The figure shows three views and two pictorial views of one solid part (mm, origin at its lowest corner). Answer the questions. A direction names the side the tool comes from. Give positions to 0.01 mm unless a question says otherwise; leave off trailing zeros. Order: outer loops, then holes, each group sorted by start corner. A loop starts at its lowest first (then second) coordinate and runs counter-clockwise, first axis right, second up. Notation, with made-up numbers: (-23.5, 23.25) - (5.5, 23.25) arc R19 cw to (5.5, 57.25) - close; hole circle Ø2 at (-22, 21). An arc over 180 degrees is marked (long way). Use a Markdown table: item, result. Add a question column.
1. Which of the six approach directions +Z, -Z, +X, -X, +Y, -Y give full straight-line access (tool end or side, diameter ignored) to the marked faces 4 and 5?
2. A cutting plane is placed at B-B on z = 154. Determine the outline of the cut face in (x, y), and give its area (3 significant figures).
3. A cutting plane is placed at A-A on x = 100. Determine the outline of the cut face in (y, z).
4. Flat-ended cylindrical pins translate along their axes: P1, Ø15, axis at x = 100, y = 330, coming from the +Z side; P2, Ø22.5, axis at x = 580, y = 50, coming from the -Z side. Find the tip coordinate at first contact, or state that the pin passes through.
5. For a pull along Z with two mould halves and no side action, classify the marked faces 1, 2 and 3 as released by +Z, released by -Z, zero draft, split by the parting line, or undercut.
6. Consider L1, parallel to Y at x = 100, z = 7; L2, parallel to Y at x = 340, z = 370; L3, parallel to Z at x = 312, y = 213.5. Determine where each line is inside the solid, lowest interval first.
7. A cutting plane is placed at C-C on y = 286.5. Determine the outline of the cut face in (x, z), and give its area (3 significant figures).
8. A cutting plane is placed at D-D on x = 204.5. Determine the outline of the cut face in (y, z).
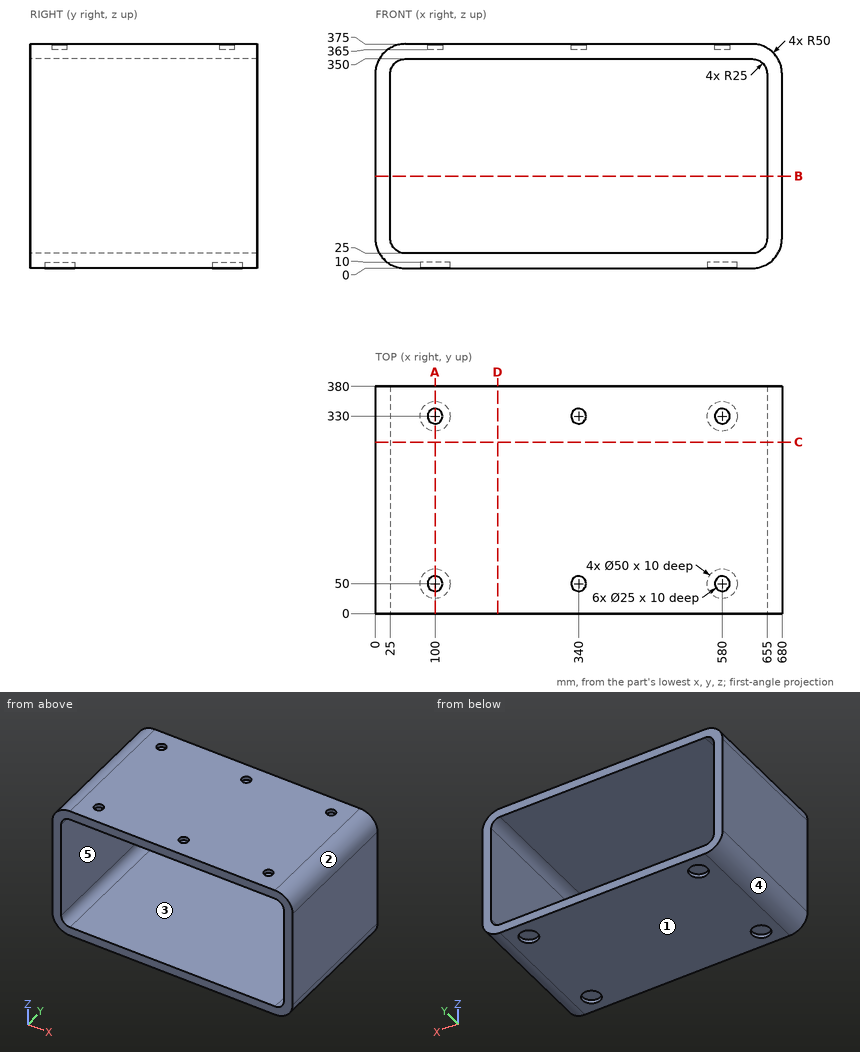
Output values:
| question | item | result |
|---|---|---|
| 1 | face 4 | -Z, -X, +Y, -Y |
| 1 | face 5 | +Y, -Y |
| 2 | outline | (0, 0) - (25, 0) - (25, 380) - (0, 380) - close; (655, 0) - (680, 0) - (680, 380) - (655, 380) - close |
| 2 | area | 19,000 mm² |
| 3 | outline | (0, 0) - (25, 0) - (25, 10) - (75, 10) - (75, 0) - (305, 0) - (305, 10) - (355, 10) - (355, 0) - (380, 0) - (380, 25) - (0, 25) - close; (0, 350) - (380, 350) - (380, 375) - (342.5, 375) - (342.5, 365) - (317.5, 365) - (317.5, 375) - (62.5, 375) - (62.5, 365) - (37.5, 365) - (37.5, 375) - (0, 375) - close |
| 4 | P1 | z = 365 |
| 4 | P2 | z = 10 |
| 5 | face 1 | released by -Z |
| 5 | face 2 | released by +Z |
| 5 | face 3 | undercut |
| 6 | L1 | 0 to 25, 75 to 305, 355 to 380 |
| 6 | L2 | 0 to 37.5, 62.5 to 317.5, 342.5 to 380 |
| 6 | L3 | 0 to 25, 350 to 375 |
| 7 | outline | (0, 50) arc R50 ccw to (50, 0) - (630, 0) arc R50 ccw to (680, 50) - (680, 325) arc R50 ccw to (630, 375) - (50, 375) arc R50 ccw to (0, 325) - close; hole (25, 50) arc R25 ccw to (50, 25) - (630, 25) arc R25 ccw to (655, 50) - (655, 325) arc R25 ccw to (630, 350) - (50, 350) arc R25 ccw to (25, 325) - close |
| 7 | area | 48,600 mm² |
| 8 | outline | (0, 0) - (380, 0) - (380, 25) - (0, 25) - close; (0, 350) - (380, 350) - (380, 375) - (0, 375) - close |
